Part model, mm, in its own coordinate system. Face numbers are marked on the shaded views. Coordinates: 2 decimals unless noted, no trailing zeros. Loops run counter-clockwise (first coordinate to the right, second up) from the corner with the lowest first, then second, coordinate; pieces in that order, holes last. Notation, with made-up numbers: (40.5, 36.5) - (89.5, 36.5) arc R14 ccw to (89.5, 44.5) - close; hole circle Ø7 at (11.25, -11.5). An arc over 180 degrees is marked (long way). Use a Markdown table: item, result. Add a question column.
1) Band-saw the part on B-B (x = -14). Give the cut face in (y, z), plus the area to 3 significant figures.
2) Drop a flat-ended pin along its axis: P1, Ø1.5, axis at x = 33, y = -44.5, coming from the -Z side. Give the stop position or say it passes through.
3) Probe probe 1 along Z at (x, y) = (6.5, -48); probe 2 along X at (y, z) = (-43, -32); probe 3 along X at (y, z) = (-50.5, 19.5). List the from-to ranges inside material, lowest first. Write a range as [from, to].
4) Pull direction X, two halves, no side cores. Call the marked faces 1, 2, 3 and 4: +X half, -X half, draft (parallel to the pull), parting line (faces both ways), or undercut.
5) Band-saw the part on A-A (y = -24). Give the cut face in (x, z).
6) Band-saw the part on C-C (z = -22). Give the cut face in (x, y), plus the area to 3 significant figures.
7) Band-saw the part on D-D (y = -35.5). Give the cut face in (x, z).
from build123d import *

# Parameters (mm, degrees)
F1_DEPTH = 60
F2_R     = 5
F3_R     = 5
F5_R     = 25
F6_DEPTH = 30
F7_R     = 25
F8_DEPTH = 30


with BuildPart() as f1:
    # F0 (on Front) → F1 (new body)
    with BuildSketch(Plane.XZ):
        with BuildLine():
            Line((28.855905, 44.195566), (-21.144095, 44.195566))
            ThreePointArc((-21.144095, 44.195566), (-38.821765, 36.873235), (-46.144095, 19.195566))
            Line((-46.144095, 19.195566), (-46.144095, 13.908361))
            Line((-46.144095, 13.908361), (-46.144095, 9.730815))
            Line((-46.144095, 9.730815), (-46.144095, -30.804434))
            ThreePointArc((-46.144095, -30.804434), (-38.821765, -48.482104), (-21.144095, -55.804434))
            Line((-21.144095, -55.804434), (28.855905, -55.804434))
            ThreePointArc((28.855905, -55.804434), (46.533574, -48.482104), (53.855905, -30.804434))
            Line((53.855905, -30.804434), (53.855905, 19.195566))
            ThreePointArc((53.855905, 19.195566), (46.533574, 36.873235), (28.855905, 44.195566))
        make_face()
    extrude(amount=F1_DEPTH)

    # F2
    f2_edges = [f1.edges().sort_by_distance(p)[0] for p in [
        (-38.821765, -60, 36.873235),
        (3.855905, -60, 44.195566),
        (-46.144095, -60, -5.804434),
        (-38.821765, -60, -48.482104),
        (3.855905, -60, -55.804434),
        (46.533574, -60, -48.482104),
        (53.855905, -60, -5.804434),
        (46.533574, -60, 36.873235),
    ]]
    fillet(f2_edges, radius=F2_R)

    # F3
    f3_edges = [f1.edges().sort_by_distance(p)[0] for p in [
        (53.855905, 0, -5.804434),
        (3.855905, 0, 44.195566),
        (-38.821765, 0, 36.873235),
        (-46.144095, 0, -5.804434),
        (-38.821765, 0, -48.482104),
        (3.855905, 0, -55.804434),
        (46.533574, 0, -48.482104),
        (46.533574, 0, 36.873235),
    ]]
    fillet(f3_edges, radius=F3_R)

    # F5 (on Front) → F6 (cut)
    with BuildSketch(Plane.XZ):
        Circle(F5_R)
    extrude(amount=-F6_DEPTH, mode=Mode.SUBTRACT)

    # F7 (on face) → F8 (cut)
    with BuildSketch(Plane.XZ.offset(60)):
        with Locations((5.336974, -6.285768)):
            Circle(F7_R)
    extrude(amount=-F8_DEPTH, mode=Mode.SUBTRACT)


solid = f1.part
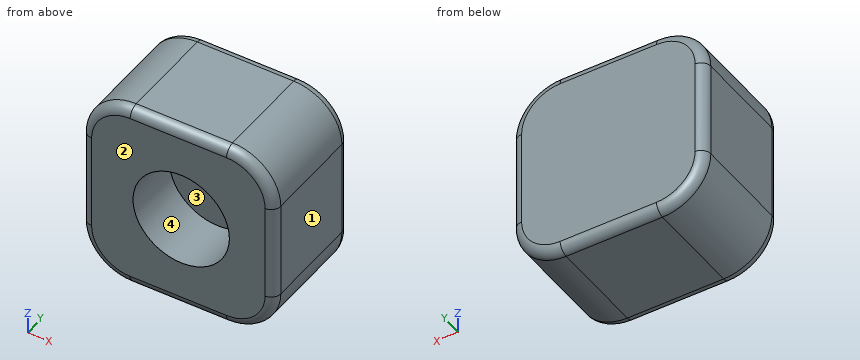
Answer block:
| question | item | result |
|---|---|---|
| 1 | outline | (-60, -50.8) arc R5 ccw to (-55, -55.8) - (-5, -55.8) arc R5 ccw to (0, -50.8) - (0, 39.2) arc R5 ccw to (-5, 44.2) - (-55, 44.2) arc R5 ccw to (-60, 39.2) - (-60, 9.56) - (-30, 9.56) - (-30, -22.13) - (-60, -22.13) - close |
| 1 | area | 5,030 mm2 |
| 2 | P1 | z = -55.57 |
| 3 | probe 1 | [-55.8, -31.26], [18.69, 44.2] |
| 3 | probe 2 | [-46.12, 53.83] |
| 3 | probe 3 | [-46.14, 53.85] |
| 4 | face 1 | +X half |
| 4 | face 2 | draft |
| 4 | face 3 | undercut |
| 4 | face 4 | undercut |
| 5 | outline | (-46.14, -30.8) arc R25 ccw to (-21.14, -55.8) - (28.86, -55.8) arc R25 ccw to (53.86, -30.8) - (53.86, 19.2) arc R25 ccw to (28.86, 44.2) - (-21.14, 44.2) arc R25 ccw to (-46.14, 19.2) - close |
| 6 | outline | (-46.14, -55) arc R5 ccw to (-41.14, -60) - (-14.11, -60) - (-14.11, -30) - (24.78, -30) - (24.78, -60) - (48.86, -60) arc R5 ccw to (53.86, -55) - (53.86, -5) arc R5 ccw to (48.86, 0) - (-41.14, 0) arc R5 ccw to (-46.14, -5) - close |
| 6 | area | 4,810 mm2 |
| 7 | outline | (-46.14, -30.8) arc R25 ccw to (-21.14, -55.8) - (28.86, -55.8) arc R25 ccw to (53.86, -30.8) - (53.86, 19.2) arc R25 ccw to (28.86, 44.2) - (-21.14, 44.2) arc R25 ccw to (-46.14, 19.2) - close; hole circle Ø50 at (5.34, -6.29) |
